```python
from build123d import *

# Parameters (mm, degrees)
SKETCH1_W           = 120
SKETCH1_H           = 100
BOSS_EXTRUDE1_DEPTH = 80
SKETCH2_W           = 40
SKETCH2_H           = 30
CUT_EXTRUDE1_DEPTH  = 80
CUT_EXTRUDE2_DEPTH  = 80
CUT_EXTRUDE6_DEPTH  = 20
SKETCH5_W           = 29.999
SKETCH5_H           = 20
CUT_EXTRUDE7_DEPTH  = 68
SKETCH6_W           = 40.001
SKETCH6_H           = 20
CUT_EXTRUDE8_DEPTH  = 68
SKETCH7_W           = 40.001
SKETCH7_H           = 20
CUT_EXTRUDE9_DEPTH  = 68
CUT_EXTRUDE10_DEPTH = 68
SKETCH13_W          = 29.999
SKETCH13_H          = 72.111025509
CUT_EXTRUDE11_DEPTH = 68
CUT_EXTRUDE12_DEPTH = 68


with BuildPart() as part:
    # Sketch1 → Boss-Extrude1 (new body)
    with BuildSketch(Plane(origin=(0, 0, 0), x_dir=(1, 0, 0), z_dir=(0, 1, 0))):
        with Locations((60, 50)):
            Rectangle(SKETCH1_W, SKETCH1_H)
    extrude(amount=BOSS_EXTRUDE1_DEPTH)

    # Sketch2 → Cut-Extrude1 (cut)
    with BuildSketch(Plane(origin=(0, 80, 0), x_dir=(1, 0, 0), z_dir=(0, 1, 0))):
        with Locations((60, 15)):
            Rectangle(SKETCH2_W, SKETCH2_H)
    extrude(amount=-CUT_EXTRUDE1_DEPTH, mode=Mode.SUBTRACT)

    # Sketch3 → Cut-Extrude2 (cut)
    with BuildSketch(Plane(origin=(0, 80, 0), x_dir=(1, 0, 0), z_dir=(0, 1, 0))):
        Polygon((0, 60), (10, 60), (10, 20), (30, 0), (0, 0), align=None)
        Polygon((120, 60), (110, 60), (110, 20), (90, 0), (120, 0), align=None)
    extrude(amount=-CUT_EXTRUDE2_DEPTH, mode=Mode.SUBTRACT)

    # Sketch4 → Cut-Extrude6 (cut)
    with BuildSketch(Plane(origin=(0, 80, 0), x_dir=(1, 0, 0), z_dir=(0, 1, 0))):
        Polygon((30, 100), (90, 100), (90, 90), (109.999, 60), (80, 60), (80, 30), (40, 30), (40, 60), (10.001, 60), (30, 90), align=None)
    extrude(amount=-CUT_EXTRUDE6_DEPTH, mode=Mode.SUBTRACT)

    # Sketch5 → Cut-Extrude7 (cut)
    with BuildSketch(Plane(origin=(0, 0, -60), x_dir=(-1, 0, 0), z_dir=(0, 0, -1))):
        with Locations((-94.9995, 70)):
            Rectangle(SKETCH5_W, SKETCH5_H)
        with Locations((-25.0005, 70)):
            Rectangle(SKETCH5_W, SKETCH5_H)
    extrude(amount=-CUT_EXTRUDE7_DEPTH, mode=Mode.SUBTRACT)

    # Sketch6 → Cut-Extrude8 (cut)
    with BuildSketch(Plane.ZY.offset(-109.999)):
        with Locations((-39.9995, 70)):
            Rectangle(SKETCH6_W, SKETCH6_H)
    extrude(amount=-CUT_EXTRUDE8_DEPTH, mode=Mode.SUBTRACT)

    # Sketch7 → Cut-Extrude9 (cut)
    with BuildSketch(Plane(origin=(10.001, 0, 0), x_dir=(0, 0, -1), z_dir=(1, 0, 0))):
        with Locations((39.9995, 70)):
            Rectangle(SKETCH7_W, SKETCH7_H)
    extrude(amount=-CUT_EXTRUDE9_DEPTH, mode=Mode.SUBTRACT)

    # Sketch10 → Cut-Extrude10 (cut)
    with BuildSketch(Plane(origin=(-5e-09, 13.846153834, 9.230769225), x_dir=(1, 0, 0), z_dir=(0, 0.832050294, 0.554700196))):
        Polygon((40.001000005, 83.205029422), (40.000000005, 11.094003927), (10.000000005, 11.094003927), (10.000000005, 83.205029436), align=None)
    extrude(amount=CUT_EXTRUDE10_DEPTH, mode=Mode.SUBTRACT)

    # Sketch13 → Cut-Extrude11 (cut)
    with BuildSketch(Plane(origin=(0, 13.846153846, 9.230769231), x_dir=(-1, 0, 0), z_dir=(0, -0.832050294, -0.554700196))):
        with Locations((-94.9995, 47.14951668)):
            Rectangle(SKETCH13_W, SKETCH13_H)
    extrude(amount=-CUT_EXTRUDE11_DEPTH, mode=Mode.SUBTRACT)

    # Sketch14 → Cut-Extrude12 (cut)
    with BuildSketch(Plane.ZY.offset(-109.999)):
        Polygon((-60, 60), (-19.999, 33.332666667), (-19.999, 60), align=None)
    extrude(amount=-CUT_EXTRUDE12_DEPTH, mode=Mode.SUBTRACT)


solid = part.part
```
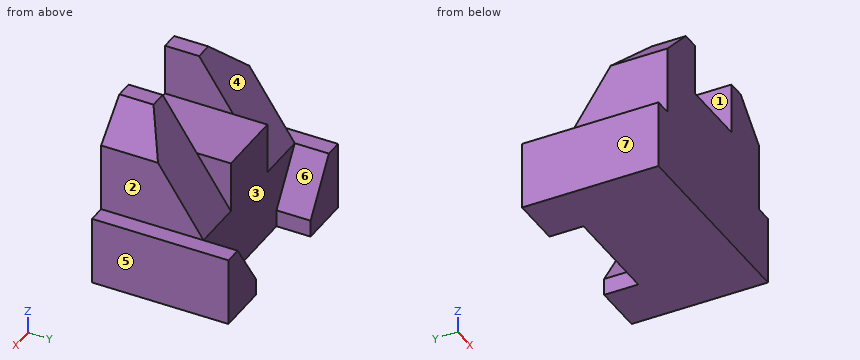
Input: part model. Units: mm. Frame: model coordinates. Face numbers are marked on the shaded views. A direction names the side the tool comes from. Give positions to 0.01 mm unless a question says otherwise; leave off trailing zeros. Write each loop counter-clockwise with the first axis right and the second up, starting at its lowest first coordinate (ties: lowest second). Pieces come first, ordered by that corner, then holes. Notation, with made-up numbers: (-2.5, -8) - (22.5, -8) arc R10 ccw to (22.5, 4) - close; hole circle Ø5 at (-6.75, 6.5). An arc over 180 degrees is marked (long way). Write item = value, one per line. Start each with the question number.
1. First-contact query: pin 1 Ø8 at (x, y) = (44.5, 46.5) entering from +Z; pin 2 Ø6 at (x, z) = (34.5, -48) entering from +Y; pin 3 Ø9 at (y, z) = (22, -20.5) entering from +X. Flat tips, straight axial feed; report the tip coordinate or a pass-through.
2. Access query for the marked faces 1, 2, 3 and 4. Directions: +Z, -Z, +X, -X, +Y, -Y. A direction counts if a zero-diameter tool reaches every point of the face in a straight line with its end or side. Return the directions, or none.
3. Ray query, L1, parallel to Z at x = 71, y = 32.5; L2, parallel to X at y = 9, z = -58.5; L3, parallel to Y at x = 31.5, z = -75. Return the intervals inside material, ascending.
4. Mould query, pull axis X, two halves, no side actions, for the marked faces 5, 6 and 7. Classes: released by +X, released by -X, zero draft, split by the parting line, or undercut.
5. Section query A-A, the plane y = 23. Output: boundary loops of the cut face in (x, z), then the cut area to 3 significant figures.
6. Section query D-D, the plane z = -81. Output: boundary loops of the cut face in (x, y).
7. Section query B-B, the plane z = -18.5. Output: boundary loops of the cut face in (x, y).
8. Section query C-C, the plane y = 63. Output: boundary loops of the cut face in (x, z), then the cut area to 3 significant figures.
Check sheet entries:
q1.pin_1 = -30
q1.pin_2 = 54
q1.pin_3 = 110
q2.face_1 = +Z, +Y, -Y
q2.face_2 = +Z, +X, +Y, -Y
q2.face_3 = +Z, +Y
q2.face_4 = +Z, -X, +Y
q3.L1 = -100 to -30
q3.L2 = 10 to 110
q3.L3 = 0 to 60
q4.face_5 = released by +X
q4.face_6 = undercut
q4.face_7 = released by -X
q5.outline = (0, -100) - (120, -100) - (120, -60) - (110, -60) - (110, -20) - (94.5, -4.5) - (80, -4.5) - (80, -30) - (40, -30) - (40, -4.5) - (25.5, -4.5) - (10, -20) - (10, -60) - (0, -60) - close
q5.area = 9,090 mm2
q6.outline = (0, 0) - (120, 0) - (120, 80) - (96, 80) - (96, 60) - (24, 60) - (24, 80) - (0, 80) - close
q7.outline = (11.5, 0) - (40, 0) - (40, 32.33) - (11.5, 32.33) - close; (80, 0) - (108.5, 0) - (108.5, 32.33) - (80, 32.33) - close
q8.outline = (0, -100) - (30, -100) - (30, -90) - (10, -60) - (0, -60) - close; (90, -100) - (120, -100) - (120, -60) - (110, -60) - (90, -90) - close
q8.area = 1,800 mm2
